Work out the finished part from the listing and answer in its coordinate system (mm). A direction names the side the tool comes from. Round coordinates to 2 decimals unless told otherwise and drop trailing zeros. Loops run counter-clockwise (first coordinate to the right, second up) from the corner with the lowest first, then second, coordinate; pieces in that order, holes last.
from build123d import *

# Parameters (mm, degrees)
F0_R      = 173.3489517692
F0_R_2    = 117.2606948697
F1_DEPTH  = 124.6887519956
F2_R      = 45.426792545
F3_R      = 121.2481204934
F4_DEPTH  = 55.2671570331
F5_R      = 75.1710071643
F6_DEPTH  = 80.0674576312
F7_R      = 32.7838298789
F8_DEPTH  = 127.7635861188
F9_R      = 21.2247552793
F11_R     = 54.14327209
F12_DEPTH = 72.1452143043
F13_R     = 16.7884886241
F14_DEPTH = 320.553438738
F15_R     = 5.7742203186
F15_R_2   = 5.0578841716
F15_R_3   = 3.8948170444
F15_R_4   = 4.1650665602
F16_DEPTH = 68.3403462172


# Not quite as in the source:
# - a fillet or chamfer that OpenCascade refuses, or shapes differently, is made with other operations: its cross-section is extruded or revolved along the edge and cut away or added


with BuildPart() as f1:
    # F0 (on Front) → F1 (new body)
    with BuildSketch(Plane.XZ):
        Circle(F0_R)
        Circle(F0_R_2, mode=Mode.SUBTRACT)
    extrude(amount=F1_DEPTH)

    # F2
    f2_edges = [f1.edges().sort_by_distance(p)[0] for p in [
        (-173.348952, 0, 0),
        (-173.348952, -124.688752, 0),
    ]]
    fillet(f2_edges, radius=F2_R)

    # F3 (on Front) → F4 (join)
    with BuildSketch(Plane.XZ):
        Circle(F3_R)
    extrude(amount=F4_DEPTH)

    # F5 (on Front) → F6 (join)
    with BuildSketch(Plane.XZ):
        Circle(F5_R)
    extrude(amount=F6_DEPTH)

    # F7 (on Front) → F8 (join)
    with BuildSketch(Plane.XZ):
        Circle(F7_R)
    extrude(amount=F8_DEPTH)

    # F9
    f9_edges = [f1.edges().sort_by_distance(p)[0] for p in [
        (-32.78383, -127.763586, 0),
    ]]
    fillet(f9_edges, radius=F9_R)

    # F10: fillet of radius 29.4120223151 on 1 edges, made by hand

    # F10_s1 → F10_t2 (revolve, cut)
    with BuildSketch(Plane.XY):
        with BuildLine():
            ThreePointArc((46.1227872623, -80.0674576312), (65.2202608468, -73.0240195216), (75.1710071643, -55.2671570331))
            Line((75.1710071643, -55.2671570331), (75.1710071643, -80.0674576312))
            Line((75.1710071643, -80.0674576312), (46.1227872623, -80.0674576312))
        make_face()
    revolve(axis=Axis((0, -80.0674576312, 0), (0, -1, 0)), mode=Mode.SUBTRACT)

    # F11 (on Front) → F12 (join)
    with BuildSketch(Plane.XZ):
        Circle(F11_R)
    extrude(amount=-F12_DEPTH)

    # F13 (on Top) → F14 (join)
    with BuildSketch(Plane.XY):
        with Locations((0, 39.3408536911)):
            Circle(F13_R)
    extrude(amount=F14_DEPTH)

    # F15 (on Front) → F16 (join)
    with BuildSketch(Plane.XZ):
        with Locations((0, 98.4903275967)):
            Circle(F15_R)
        with Locations((-93.0983424187, 0)):
            Circle(F15_R_2)
        with Locations((0, -94.7722494602)):
            Circle(F15_R_3)
        with Locations((95.7255959511, 0)):
            Circle(F15_R_4)
    extrude(amount=F16_DEPTH)


solid = f1.part
Item 1: Each of these flat-tipped pins is pushed along its axis until it touches: P1, Ø6, axis at x = 19, y = -25.5, coming from the -Z side; P2, Ø11, axis at x = -95.5, z = 0, coming from the -Y side; P3, Ø3, axis at x = 16.5, y = -49, coming from the -Z side. Where does it stop, or does it pass through?
Item 2: For faces 4 (the face through (-86.426, -89.492, 79.25)), 5 (the face through (-1, 72.145, 1)), determine the directions among +Z, -Z, +X, -X, +Y, -Y from which every point of the face is accessible in a straight line to the end or side of a thin tool.
Item 3: Straight lines are drawn through the part: line 1 (Z direction, x = 0, y = -71); line 2 (Z direction, x = 0, y = -96.5); line 3 (Y direction, x = -29.5, z = 93). For each, find the intervals that lie inside material, in ascending order.
Item 4: Section B-B, the plane y = -13.5 is taken. Give the vertices of the cut face in (x, z), plus the area to 3 significant figures.
Item 5: Determine the mould class of faces 1 (the face through (-11.737, 35.568, -52.856)), 2 (the face through (-98.15, -61.71, 0.22)), 3 (the face through (-3.64, 22.95, 184.13)) for opening direction Z: pulls with the +Z half, pulls with the -Z half, needs draft (parallel to the pull), parting line crosses it, or undercut.
Item 6: Section A-A, the plane z = 204 is taken. Give the vertices of the cut face in (x, y).
Answer below:
1. P1: stops at z = -169.06
1. P2: stops at y = -68.34
1. P3: stops at z = -172.7
2. face 4: -Y
2. face 5: +Z, -Z, +X, -X, +Y
3. line 1: z = -173.35 to -117.26, -67.36 to 67.36, 117.26 to 173.35
3. line 2: z = -169.95 to -117.26, -32.78 to 32.78, 117.26 to 169.95
3. line 3: y = -55.27 to 0
4. outline: circle Ø320.47 at (0, 0)
4. area: 80,700 mm2
5. face 1: parting line crosses it
5. face 2: undercut
5. face 3: needs draft
6. outline: circle Ø33.58 at (0, 39.34)
